Design review of the part built by this model. Coordinates are the model's own, in mm. A direction names the side the tool comes from. Round coordinates to 2 decimals unless told otherwise and drop trailing zeros. Order: outer loops, then holes, each group sorted by start corner. A loop starts at its lowest first (then second) coordinate and runs counter-clockwise, first axis right, second up. Notation, with made-up numbers: (52, 0.25) - (58, 0.25) arc R12 ccw to (58, 22.25) - close; hole circle Ø11 at (11.25, 84.25). An arc over 180 degrees is marked (long way). Write item = value, one per line.
from build123d import *

# Parameters (mm, degrees)
SKETCH1_R                = 27.051
SKETCH1_R_2              = 19.8628
EXTRUDE1_DEPTH           = 7.9248
CHAMFER1_SIZE            = 0.567944
CHAMFER2_SIZE            = 1.0922
CUT_EXTRUDE1_DEPTH       = 8.9248
FILLET1_R                = 0.4064
CIRPATTERN1_COUNT        = 4
FILLET1_OF_CIRPATTERN1_R = 0.4064


with BuildPart() as part:
    # Sketch1 → Extrude1 (new body)
    with BuildSketch(Plane.XY):
        Circle(SKETCH1_R)
        Circle(SKETCH1_R_2, mode=Mode.SUBTRACT)
    extrude(amount=EXTRUDE1_DEPTH)

    # Chamfer1
    chamfer1_edges = [part.edges().sort_by_distance(p)[0] for p in [
        (-27.051, 0, 0),
        (-27.051, 0, 7.9248),
    ]]
    chamfer(chamfer1_edges, length=CHAMFER1_SIZE)

    # Chamfer2
    chamfer2_edges = [part.edges().sort_by_distance(p)[0] for p in [
        (-19.8628, 0, 0),
        (-19.8628, 0, 7.9248),
    ]]
    chamfer(chamfer2_edges, length=CHAMFER2_SIZE)

    # Sketch2 → Cut-Extrude1 (cut, through all)
    with BuildSketch(Plane.XY.offset(7.9248)):
        with BuildLine():
            Line((16.750672018, 21.240800078), (15.014988234, 19.505116295))
            Line((15.014988234, 19.505116295), (19.505116295, 15.014988234))
            Line((19.505116295, 15.014988234), (21.240800078, 16.750672018))
            ThreePointArc((21.240800078, 16.750672018), (19.127945538, 19.127945538), (16.750672018, 21.240800078))
        make_face()
    cut_extrude1 = extrude(amount=-CUT_EXTRUDE1_DEPTH, mode=Mode.SUBTRACT)

    # Fillet1
    fillet1_edges = [part.edges().sort_by_distance(p)[0] for p in [
        (19.505116295, 15.014988234, 3.9624),
        (15.014988234, 19.505116295, 3.9624),
    ]]
    fillet(fillet1_edges, radius=FILLET1_R)

    # CirPattern1: Cut-Extrude1 ×4 about axis
    cirpattern1_axis = Axis((0, 0, 0), (0, 0, 1))
    for i in range(1, CIRPATTERN1_COUNT):
        add(cut_extrude1.rotate(cirpattern1_axis, i * 360 / CIRPATTERN1_COUNT), mode=Mode.SUBTRACT)

    # Fillet1 of CirPattern1
    fillet1_of_cirpattern1_edges = [part.edges().sort_by_distance(p)[0] for p in [
        (-15.014988234, 19.505116295, 3.9624),
        (-19.505116295, 15.014988234, 3.9624),
        (-19.505116295, -15.014988234, 3.9624),
        (-15.014988234, -19.505116295, 3.9624),
        (15.014988234, -19.505116295, 3.9624),
        (19.505116295, -15.014988234, 3.9624),
    ]]
    fillet(fillet1_of_cirpattern1_edges, radius=FILLET1_OF_CIRPATTERN1_R)


solid = part.part
Item 1: For faces 1 (the face through (17.23, 17.29, 4.02)), 2 (the face through (-20.51, -16.02, 4.02)), 3 (the face through (-18, -12, 7.925)), 4 (the face through (20.51, 16.02, 4.02)), list the 3-axis set-ups (+Z, -Z, +X, -X, +Y, -Y) from which the entire face can be reached by the end or side of a thin tool; tool diameter is ignored.
Data:
face_1 = +Z, -Z
face_2 = +Z, -Z, -Y
face_3 = +Z, +X, -X, +Y, -Y
face_4 = +Z, -Z, +Y
Item 2: The part is to be moulded in two halves that separate along Y. For faces 5 (the face through (-27.05, 0.25, 3.91)), 6 (the face through (-17.29, 17.23, 4.02)), 7 (the face through (-0.25, -27.05, 3.91)), 8 (the face through (-16.04, -20.53, 4.02)), say which applies: +Y half, -Y half, draft (parallel to the pull), parting line (faces both ways), or undercut.
Data:
face_5 = parting line
face_6 = undercut
face_7 = -Y half
face_8 = undercut
Item 3: Take a section at C-C, the plane z = 3. State the section outline as (x, y) points, and give its area (3 significant figures).
Data:
outline = (-21.24, -16.75) - (-19.79, -15.3) arc R0.41 cw to (-19.22, -15.3) - (-15.3, -19.22) arc R0.41 cw to (-15.3, -19.79) - (-16.75, -21.24) arc R27.05 ccw to (16.75, -21.24) - (15.3, -19.79) arc R0.41 cw to (15.3, -19.22) - (19.22, -15.3) arc R0.41 cw to (19.79, -15.3) - (21.24, -16.75) arc R27.05 ccw to (21.24, 16.75) - (19.79, 15.3) arc R0.41 cw to (19.22, 15.3) - (15.3, 19.22) arc R0.41 cw to (15.3, 19.79) - (16.75, 21.24) arc R27.05 ccw to (-16.75, 21.24) - (-15.3, 19.79) arc R0.41 cw to (-15.3, 19.22) - (-19.22, 15.3) arc R0.41 cw to (-19.79, 15.3) - (-21.24, 16.75) arc R27.05 ccw to start; hole circle Ø39.73 at (0, 0)
area = 994 mm2
Item 4: For line 1 along Y through (x, z) = (0, 5.5); line 2 along X through (y, z) = (12.5, 6); line 3 along X through (y, z) = (6.5, 5.5), list the stretches that pass through material, from the lowest coordinate up. Write a range as [from, to].
Data:
line_1 = [-27.05, -19.86], [19.86, 27.05]
line_2 = [-23.99, -15.44], [15.44, 23.99]
line_3 = [-26.26, -18.77], [18.77, 26.26]
Item 5: Take a section at A-A, the plane y = 0. State the section outline as (x, z) points (3 decimals).
Data:
outline = (-27.051, 0.568) - (-26.483, 0) - (-20.955, 0) - (-19.863, 1.092) - (-19.863, 6.833) - (-20.955, 7.925) - (-26.483, 7.925) - (-27.051, 7.357) - close; (19.863, 1.092) - (20.955, 0) - (26.483, 0) - (27.051, 0.568) - (27.051, 7.357) - (26.483, 7.925) - (20.955, 7.925) - (19.863, 6.833) - close
Item 6: Insertion check: P1, Ø1.5, axis at x = -21, z = 3, coming from the +Y side; P2, Ø3, axis at y = 13, z = 6.5, coming from the -X side; P3, Ø4, axis at x = 8, z = 6, coming from the -Y side. Each pin has a flat end and moves straight along its axis. Give the tip position at first contact, or say it passes through.
Data:
P1 = 16.75
P2 = -24.48
P3 = -26.38
